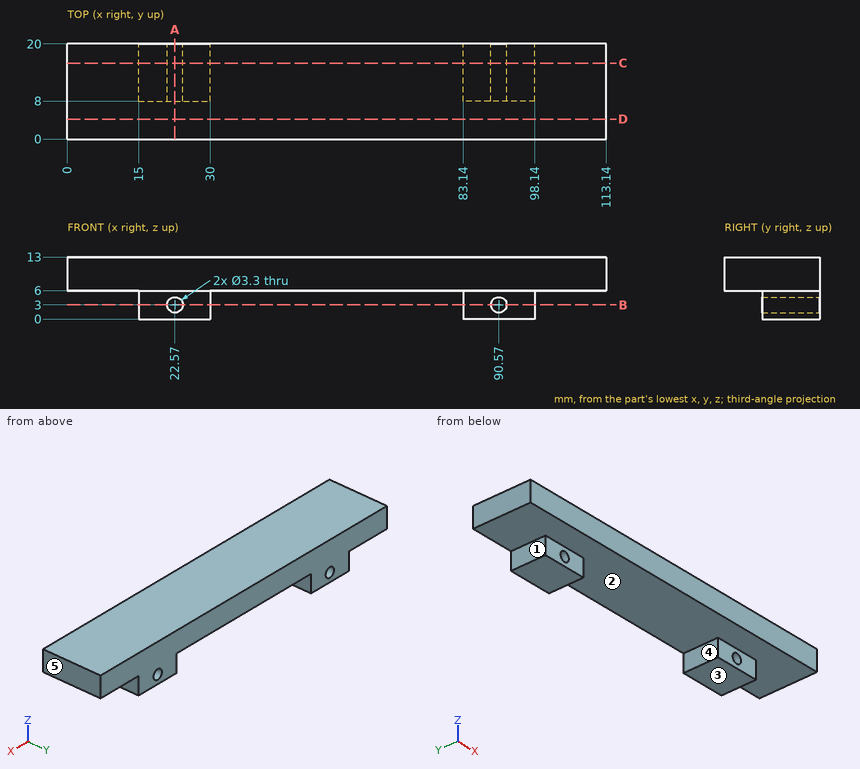
Geometry: see drawing. Coordinates: mm, zero at the bounding-box minimum. A direction names the side the tool comes from. Round coordinates to 2 decimals unless told otherwise and drop trailing zeros. Write each loop counter-clockwise with the first axis right and the second up, starting at its lowest first coordinate (ties: lowest second). Pieces come first, ordered by that corner, then holes. Notation, with made-up numbers: M 20.25,-29.5 L 53.25,-29.5 A23 ccw 53.25,0.5 Z; hole C -27,74 d3. An arc over 180 degrees is marked long. Answer as a JSON object with one key per item and string values. Group by question number.
(1) Reachability of the marked faces 4 and 5 from +Z, -Z, +X, -X, +Y, -Y: full face, straight path, thin tool, end or side. Return the list, or none.
(2) Ray query, line 1 (X direction, y = 14.25, z = 3); line 2 (X direction, y = 18, z = 1.5); line 3 (Z direction, x = 22.57, y = 13.5). Return the intervals inside material, ascending. Write a range as [from, to].
(3) Section query C-C on y = 16. Output: boundary loops of the cut face in (x, z), then the cut area to 3 significant figures.
(4) Section query A-A on x = 22.57. Output: boundary loops of the cut face in (y, z).
(5) Mould query, pull axis X, two halves, no side actions, for the marked faces 1, 2 and 3. Classes: +X half, -X half, draft (parallel to the pull), parting line (faces both ways), or undercut.
(6) First-contact query: pin 1 (5 mm diameter, centred on y = 16, z = 1.5, fed in from -X); pin 2 (2 mm diameter, centred on x = 90.57, z = 3, fed in from +Y); pin 3 (5 mm diameter, centred on y = 7.5, z = 7, fed in from -X); pin 4 (10 mm diameter, centred on x = 54, y = 11, fed in from -Z). Flat tips, straight axial feed; report the tip coordinate or a pass-through.
(7) Section query D-D on y = 4.25. Output: boundary loops of the cut face in (x, z), then the cut area to 3 significant figures.
(8) Section query B-B on z = 3. Output: boundary loops of the cut face in (x, y), then the cut area to 3 significant figures.
Computed values:
{
 "1": {"face 4": "-Z, +Y, -Y", "face 5": "+Z, -Z, +X, +Y, -Y"},
 "2": {"line 1": "[15, 20.92], [24.22, 30], [83.14, 88.92], [92.22, 98.14]", "line 2": "[15, 21.88], [23.26, 30], [83.14, 89.88], [91.26, 98.14]", "line 3": "[0, 1.35], [4.65, 13]"},
 "3": {"outline": "M 0,6 L 15,6 L 15,0 L 30,0 L 30,6 L 83.14,6 L 83.14,0 L 98.14,0 L 98.14,6 L 113.14,6 L 113.14,13 L 0,13 Z; hole C 22.57,3 d3.3; hole C 90.57,3 d3.3", "area": "955 mm^2"},
 "4": {"outline": "M 0,6 L 8,6 L 8,4.65 L 20,4.65 L 20,13 L 0,13 Z; M 8,0 L 20,0 L 20,1.35 L 8,1.35 Z"},
 "5": {"face 1": "-X half", "face 2": "undercut", "face 3": "draft"},
 "6": {"pin 1": "x = 15", "pin 2": "through", "pin 3": "x = 0", "pin 4": "z = 6"},
 "7": {"outline": "M 0,6 L 113.14,6 L 113.14,13 L 0,13 Z", "area": "792 mm^2"},
 "8": {"outline": "M 15,8 L 20.92,8 L 20.92,20 L 15,20 Z; M 24.22,8 L 30,8 L 30,20 L 24.22,20 Z; M 83.14,8 L 88.92,8 L 88.92,20 L 83.14,20 Z; M 92.22,8 L 98.14,8 L 98.14,20 L 92.22,20 Z", "area": "281 mm^2"}
}
